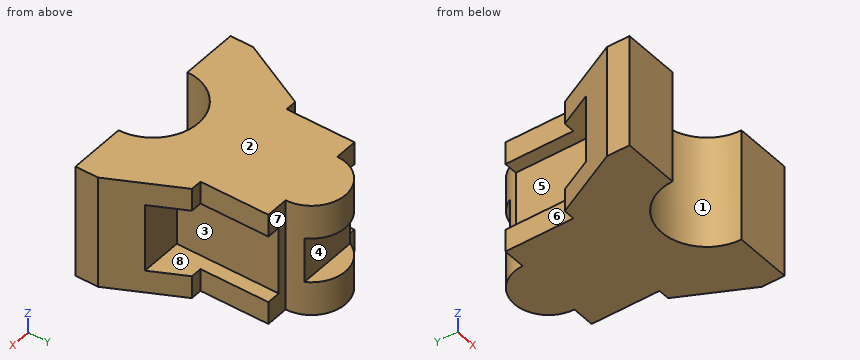
from build123d import *

# Parameters (mm, degrees)
BOSS_EXTRUDE2_DEPTH = 25
SKETCH6_W           = 20
SKETCH6_H           = 8
CUT_EXTRUDE1_DEPTH  = 25
CUT_EXTRUDE2_DEPTH  = 51
SKETCH11_W          = 26
SKETCH11_H          = 30
CUT_EXTRUDE3_DEPTH  = 45


with BuildPart() as part:
    # Sketch3 → Boss-Extrude2 (new body, symmetric)
    with BuildSketch(Plane.XY):
        with BuildLine():
            Line((0, 85), (0, 70))
            Line((0, 70), (15, 70))
            ThreePointArc((15, 70), (10.606601718, 80.606601718), (0, 85))
        make_face()
        with BuildLine():
            Line((-15, 70), (0, 70))
            Line((0, 70), (0, 85))
            ThreePointArc((0, 85), (-10.606601718, 80.606601718), (-15, 70))
        make_face()
        Polygon((0, 70), (0, 40), (25, 40), (25, 70), (15, 70), align=None)
        Polygon((-45, 0), (0, 0), (0, 40), (-25, 40), (-30, 40), (-45, 10), align=None)
        Polygon((0, 0), (45, 0), (45, 10), (30, 40), (25, 40), (0, 40), align=None)
        Polygon((-25, 40), (0, 40), (0, 70), (-15, 70), (-25, 70), align=None)
    extrude(amount=BOSS_EXTRUDE2_DEPTH, both=True)

    # Sketch6 → Cut-Extrude1 (cut, symmetric)
    with BuildSketch(Plane(origin=(0, 0, 0), x_dir=(0, 0, -1), z_dir=(1, 0, 0))):
        with Locations((0, 81)):
            Rectangle(SKETCH6_W, SKETCH6_H)
    extrude(amount=CUT_EXTRUDE1_DEPTH, both=True, mode=Mode.SUBTRACT)

    # Sketch7 → Cut-Extrude2 (cut, through all)
    with BuildSketch(Plane(origin=(0, 0, -25), x_dir=(-1, 0, 0), z_dir=(0, 0, -1))):
        with BuildLine():
            Line((-20, 0), (20, 0))
            ThreePointArc((20, 0), (0, 20), (-20, 0))
        make_face()
    extrude(amount=-CUT_EXTRUDE2_DEPTH, mode=Mode.SUBTRACT)

    # Sketch11 → Cut-Extrude3 (cut)
    with BuildSketch(Plane(origin=(0, 70, 0), x_dir=(1, 0, 0), z_dir=(0, 1, 0))):
        with Locations((-32, 0)):
            Rectangle(SKETCH11_W, SKETCH11_H)
        with Locations((32, 0)):
            Rectangle(SKETCH11_W, SKETCH11_H)
    extrude(amount=-CUT_EXTRUDE3_DEPTH, mode=Mode.SUBTRACT)


solid = part.part
Check sheet for the modelled part. Datum: model origin and axes. Units: mm. Face numbers are marked on the shaded views. A direction names the side the tool comes from. Round coordinates to 2 decimals unless told otherwise and drop trailing zeros. Order: outer loops, then holes, each group sorted by start corner. A loop starts at its lowest first (then second) coordinate and runs counter-clockwise, first axis right, second up.
(1) Cross-section at C-C, the plane x = 0. Enter the section's corners in (y, z).
(2) Cross-section at B-B, the plane y = 34. Enter the section's corners in (x, z).
(3) Access from +Z, -Z, +X, -X, +Y, -Y to the whole of each face (thin tool, end or side, straight path). Record for the marked faces 5, 6, 7 and 8.
(4) Go/stop test with flat-tipped pins: P1, Ø2, axis at y = 47, z = 19.5, coming from the -X side; P2, Ø6, axis at y = 32, z = 3.5, coming from the +X side; P3, Ø11, axis at y = 52.5, z = 21, coming from the +X side. Record where each tip stops, or that it passes through.
(5) Scan lines: probe 1 along X at (y, z) = (25.5, -11.5); probe 2 along X at (y, z) = (55, 23); probe 3 along Z at (x, y) = (-8, 81.5). Record each from-to range of solid material in increasing order.
(6) Draft check along Z on the marked faces 1, 2, 3 and 4. Enter one of: pulls with the +Z half, pulls with the -Z half, needs draft (parallel to the pull), parting line crosses it, or undercut.
(7) Cross-section at D-D, the plane y = 13. Enter the section's corners in (x, z), and give its area (3 significant figures).
(8) Cross-section at A-A, the plane z = -16.5. Enter the section's corners in (x, y), and give its area (3 significant figures).
Check sheet entries:
1. outline: (20, -25) - (85, -25) - (85, -10) - (77, -10) - (77, 10) - (85, 10) - (85, 25) - (20, 25) - close
2. outline: (-33, -25) - (33, -25) - (33, -15) - (19, -15) - (19, 15) - (33, 15) - (33, 25) - (-33, 25) - (-33, 15) - (-19, 15) - (-19, -15) - (-33, -15) - close
3. face 5: -X, +Y
3. face 6: +Z, -Z, -X, +Y
3. face 7: +Z, -Z, +X, +Y
3. face 8: +X, +Y
4. P1: stops at x = -25
4. P2: stops at x = 19
4. P3: stops at x = 25
5. probe 1: x = -19 to 19
5. probe 2: x = -25 to 25
5. probe 3: z = -25 to -10, 10 to 25
6. face 1: needs draft
6. face 2: pulls with the +Z half
6. face 3: undercut
6. face 4: undercut
7. outline: (-43.5, -25) - (-15.2, -25) - (-15.2, 25) - (-43.5, 25) - close; (15.2, -25) - (43.5, -25) - (43.5, 25) - (15.2, 25) - close
7. area: 2,830 mm2
8. outline: (-45, 0) - (-20, 0) arc R20 cw to (20, 0) - (45, 0) - (45, 10) - (30, 40) - (25, 40) - (25, 70) - (15, 70) arc R15 ccw to (-15, 70) - (-25, 70) - (-25, 40) - (-30, 40) - (-45, 10) - close
8. area: 4,380 mm2
